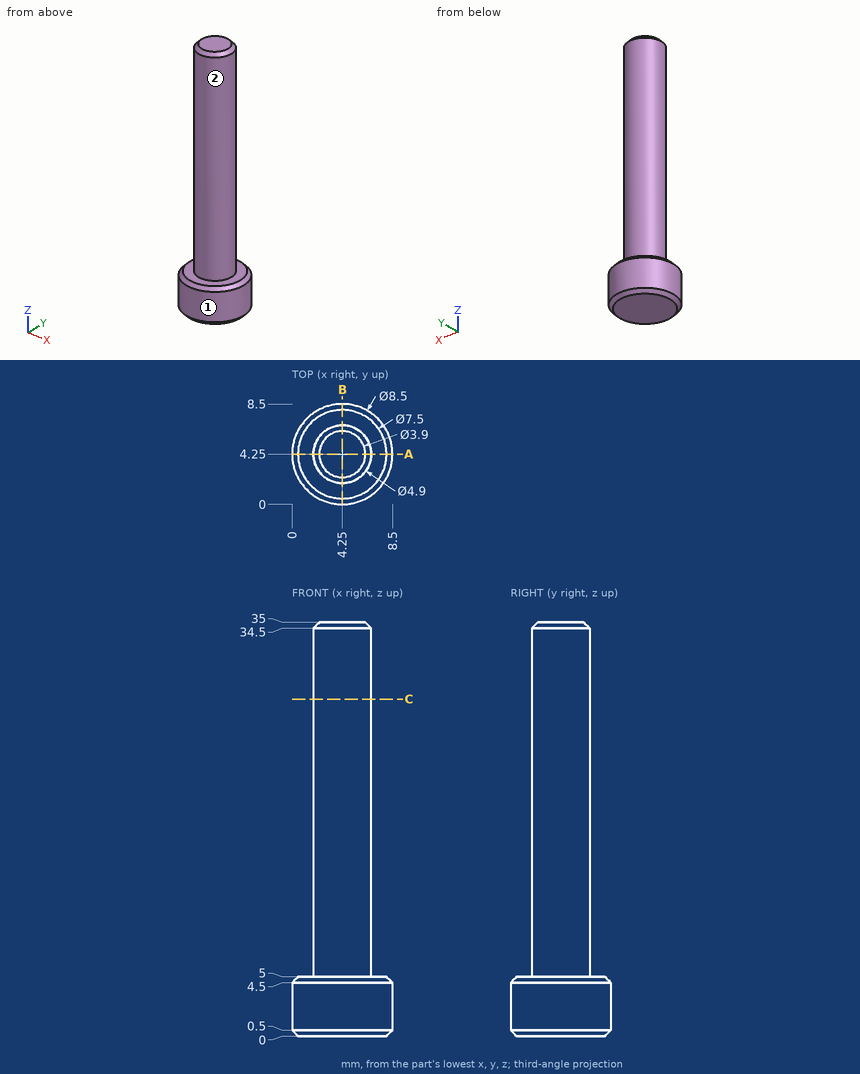
The figure shows three views and two pictorial views of one solid part (mm, origin at its lowest corner). Answer the questions. A direction names the side the tool comes from. Give positions to 0.01 mm unless a question says otherwise; leave off trailing zeros. Loops run counter-clockwise (first coordinate to the right, second up) from the corner with the lowest first, then second, coordinate; pieces in that order, holes last. Notation, with made-up numbers: (85, 86) - (89, 86) arc R23 cw to (89, 96) - close; hole circle Ø2 at (-12, -3). An arc over 180 degrees is marked (long way). Answer in a Markdown table with one row per item.
(1) Consider L1, parallel to Z at x = 1, y = 3; L2, parallel to X at y = 4.25, z = 29.5; L3, parallel to X at y = 2.75, z = 26. Determine where each line is inside the solid, lowest interval first. Write a range as [from, to].
Results list:
| item | result |
|---|---|
| L1 | z = [0, 5] |
| L2 | x = [1.8, 6.7] |
| L3 | x = [2.31, 6.19] |
(2) A tool of negligible diameter and unlimited length cuts with its end or side. For the marked faces 1 and 2, from which of +Z, -Z, +X, -X, +Y, -Y can it reach the whole face along a straight path? Write none if from no direction.
Results list:
| item | result |
|---|---|
| face 1 | +Z, -Z |
| face 2 | +Z |
(3) Section A-A (y = 4.25) is taken. Give the vertices of the cut face in (x, z).
Results list:
| item | result |
|---|---|
| outline | (0, 0.5) - (0.5, 0) - (8, 0) - (8.5, 0.5) - (8.5, 4.5) - (8, 5) - (6.7, 5) - (6.7, 34.5) - (6.2, 35) - (2.3, 35) - (1.8, 34.5) - (1.8, 5) - (0.5, 5) - (0, 4.5) - close |
(4) Flat-ended cylindrical pins translate along their axes: pin 1 Ø1.5 at (x, z) = (5, 21) entering from +Y; pin 2 Ø5 at (y, z) = (2, 6.5) entering from -X; pin 3 Ø2 at (y, z) = (1.5, 23.5) entering from -X. Find the tip coordinate at first contact, or state that the pin passes through.
Results list:
| item | result |
|---|---|
| pin 1 | stops at y = 6.7 |
| pin 2 | stops at x = 0.07 |
| pin 3 | stops at x = 2.54 |
(5) Section C-C (z = 28.5) is taken. Give the vertices of the cut face in (x, y).
Results list:
| item | result |
|---|---|
| outline | circle Ø4.9 at (4.25, 4.25) |
